```python
from build123d import *

# Parameters (mm, degrees)
F2_R           = 17.4244
F3_DEPTH       = 101.6
F5_D           = 9.525
F5_CBORE_D     = 19.05
F5_CBORE_DEPTH = 7.62
F7_DEPTH       = 838.2
F8_R           = 5.08


with BuildPart() as f1:
    # F0 (on Front) → F1 (revolve)
    with BuildSketch(Plane.XZ):
        Polygon((25.4, -38.654042), (25.4, 27.893958), (0, 27.893958), (0, -22.906042), (-34.925, -22.906042), (-34.925, -38.654042), align=None)
    revolve(axis=Axis((25.4, 0, -5.380042), (0, 0, -1)))

    # F2 (on face) → F3 (cut)
    with BuildSketch(Plane.XY.offset(27.893958)):
        with Locations((25.4, 0)):
            Circle(F2_R)
    extrude(amount=-F3_DEPTH, mode=Mode.SUBTRACT)

    # F5 (through all)
    with Locations(Plane.XY.offset(-22.906042)):
        with Locations((-17.526, 0), (25.4, -42.926), (68.326, 0)):
            CounterBoreHole(F5_D / 2, F5_CBORE_D / 2, F5_CBORE_DEPTH)

    # F6 (on face) → F7 (cut)
    with BuildSketch(Plane.XY.offset(27.893958)):
        with BuildLine():
            Line((11.176, 0), (39.624, 0))
            Line((39.624, 0), (39.624, 31.496))
            Line((39.624, 31.496), (31.490646, 31.496))
            Line((31.490646, 31.496), (31.490646, 42.67057))
            ThreePointArc((31.490646, 42.67057), (25.4, 49.022), (19.309354, 42.67057))
            Line((19.309354, 42.67057), (19.309354, 31.496))
            Line((19.309354, 31.496), (11.176, 31.496))
            Line((11.176, 31.496), (11.176, 0))
        make_face()
    extrude(amount=-F7_DEPTH, mode=Mode.SUBTRACT)

    # F8
    f8_edges = [f1.edges().sort_by_distance(p)[0] for p in [
        (11.176, 31.496, -30.780042),
        (39.624, 31.496, -30.780042),
    ]]
    fillet(f8_edges, radius=F8_R)


solid = f1.part
```
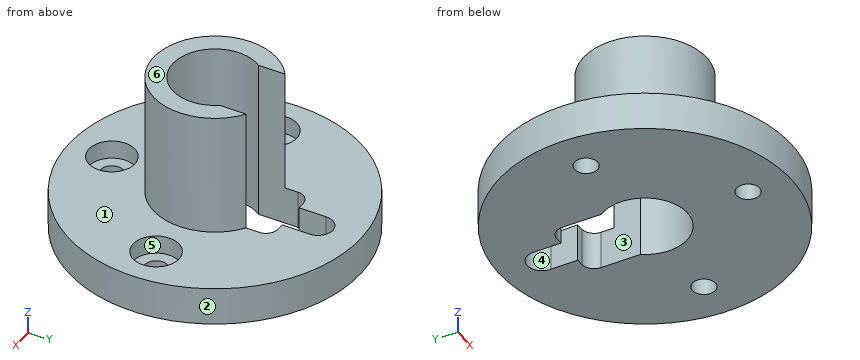
Here's how the part is built. I have some questions about the finished solid (model axes, mm). Face numbers are marked on the shaded views. A direction names the side the tool comes from. Coordinates: 2 decimals unless noted, no trailing zeros. Write each loop counter-clockwise with the first axis right and the second up, starting at its lowest first coordinate (ties: lowest second). Pieces come first, ordered by that corner, then holes. Notation, with made-up numbers: M -22.5,2.5 L 4.5,2.5 A34 ccw 4.5,36.5 Z; hole C 88.5,82 d5. An arc over 180 degrees is marked long. Answer as CSV lines item,"result". Start each with the question number.
Q1. Suppose I cut it at C-C, the plane y = -44.5. List the corners of the cut face in (x, z) for me, then the cut area to 3 significant figures.
Q2. Suppose I cut it at B-B, the plane x = 25.4. List the corners of the cut face in (y, z) for me (1 decimal), then the cut area to 3 significant figures.
Q3. Suppose I cut it at D-D, the plane x = -20. List the corners of the cut face in (y, z) for me, then the cut area to 3 significant figures.
Q4. Will these pins go through, and if not, where does the flat tip stop? pin 1 Ø15 at (x, y) = (-18.5, 2.5) entering from +Z; pin 2 Ø13 at (y, z) = (19, 8) entering from +X; pin 3 Ø5.5 at (x, y) = (70, 1.5) entering from +Z.
Q5. If we mould it in two halves opening along X, with no side actions, what happens to the marked faces 1, 2 and 3? For each: pulls with the +X half, pulls with the -X half, needs draft (parallel to the pull), parting line crosses it, or undercut.
Q6. For the marked faces 4, 5 and 6, which set-ups out of +Z, -Z, +X, -X, +Y, -Y let a thin tool reach every point of the face, with its end or its side?
Q7. Suppose I cut it at A-A, the plane y = 0. List the corners of the cut face in (x, z) for me (1 decimal).
Q8. I need wall thicknesses on probe 1 along X at (y, z) = (0, 14); probe 2 along Z at (x, y) = (-16.5, -26.5); probe 3 along Z at (x, y) = (32.5, -46). Which ranges of each line are inside material? Lowest first, please. Write a range as [from, to].
Entries:
1,outline,"M -15.33,-38.65 L 20.91,-38.65 L 20.91,-30.53 L 16.01,-30.53 L 16.01,-22.91 L -15.33,-22.91 Z; M 29.89,-38.65 L 66.13,-38.65 L 66.13,-22.91 L 34.79,-22.91 L 34.79,-30.53 L 29.89,-30.53 Z"
1,area,"1,070 mm²"
2,outline,"M -60.3,-38.7 L -47.7,-38.7 L -47.7,-30.5 L -52.5,-30.5 L -52.5,-22.9 L -60.3,-22.9 Z; M -38.2,-38.7 L -17.4,-38.7 L -17.4,27.9 L -25.4,27.9 L -25.4,-22.9 L -33.4,-22.9 L -33.4,-30.5 L -38.2,-30.5 Z; M 49,-38.7 L 60.3,-38.7 L 60.3,-22.9 L 49,-22.9 Z"
2,area,"1,040 mm²"
3,outline,"M -39.72,-38.65 L -4.07,-38.65 L -4.07,-30.53 L -9.2,-30.53 L -9.2,-22.91 L -39.72,-22.91 Z; M 4.07,-38.65 L 39.72,-38.65 L 39.72,-22.91 L 9.2,-22.91 L 9.2,-30.53 L 4.07,-30.53 Z"
3,area,"1,040 mm²"
4,pin 1,"stops at z = -22.91"
4,pin 2,"stops at x = 47.51"
4,pin 3,"stops at z = -30.53"
5,face 1,"needs draft"
5,face 2,"parting line crosses it"
5,face 3,"undercut"
6,face 4,"+Z, -Z"
6,face 5,"+Z"
6,face 6,"+Z, +X, -X, +Y, -Y"
7,outline,"M -34.9,-38.7 L -22.3,-38.7 L -22.3,-30.5 L -27.1,-30.5 L -27.1,-22.9 L -34.9,-22.9 Z; M -12.8,-38.7 L 8,-38.7 L 8,27.9 L 0,27.9 L 0,-22.9 L -8,-22.9 L -8,-30.5 L -12.8,-30.5 Z; M 42.8,-38.7 L 63.6,-38.7 L 63.6,-30.5 L 58.8,-30.5 L 58.8,-22.9 L 50.8,-22.9 L 50.8,27.9 L 42.8,27.9 Z; M 73.1,-38.7 L 85.7,-38.7 L 85.7,-22.9 L 77.9,-22.9 L 77.9,-30.5 L 73.1,-30.5 Z"
8,probe 1,"x = [0, 7.98], [42.82, 50.8]"
8,probe 2,"z = [-38.65, -22.91]"
8,probe 3,"z = [-38.65, -30.53]"
